Here's how the part is built. I have some questions about the finished solid (model axes, mm). Face numbers are marked on the shaded views. A direction names the side the tool comes from. Coordinates: 2 decimals unless noted, no trailing zeros. Order: outer loops, then holes, each group sorted by start corner. A loop starts at its lowest first (then second) coordinate and runs counter-clockwise, first axis right, second up. Notation, with made-up numbers: (60.25, 34.5) - (73.25, 34.5) arc R9 ccw to (73.25, 49.5) - close; hole circle Ø10 at (43, -8.5). An arc over 180 degrees is marked (long way). Answer as CSV lines item,"result". Start each with the question number.
Q1. For pin 1 Ø7.5 at (y, z) = (-3, 12) entering from +X; pin 2 Ø10 at (x, z) = (-19.5, 12.5) entering from +Y; pin 3 Ø2 at (x, y) = (26.5, -24) entering from +Z; pin 4 Ø2.5 at (x, z) = (4, 13) entering from -Y, each with a flat end and sliding along its axis, tell me the tip position at first contact or that it passes through.
Q2. Thinking about a two-plate mould opening in X: for the marked faces 6, 7, 8 and 9, which applies, released by +X, released by -X, zero draft, split by the parting line, or undercut?
Q3. Suppose I cut it at A-A (y = 0). Please give me the cut outline in (x, z) (3 decimals).
Q4. For the marked faces 1, 2, 3, 4 and 5, which set-ups out of +Z, -Z, +X, -X, +Y, -Y let a thin tool reach every point of the face, with its end or its side?
Q5. Suppose I cut it at B-B (z = 8.5). Please give me the cut outline in (x, y), then the cut area to 3 significant figures.
Q6. I need wall thicknesses on line 1 (X direction, y = 4, z = 5.5) (3 decimals); line 2 (X direction, y = -4, z = 12.5); line 3 (Z direction, x = -4, y = 0). Which ranges of each line are inside material? Lowest first, please.
Q7. Suppose I cut it at D-D (z = 20.5). Please give me the cut outline in (x, y).
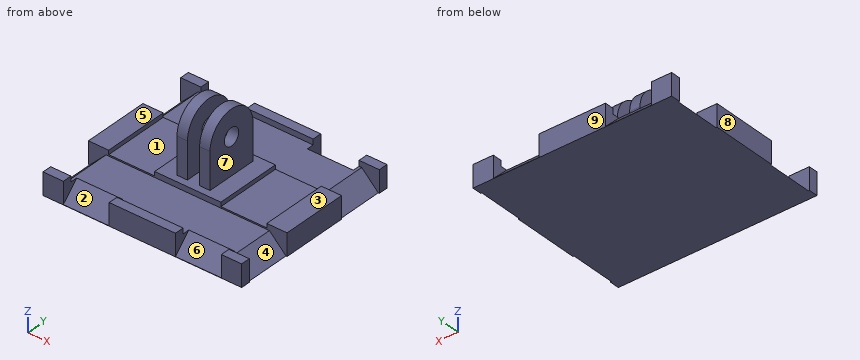
from build123d import *

# Parameters (mm, degrees)
F0_W         = 57.15
F0_H         = 50.8
F1_DEPTH     = 6.35
F2_W         = 13.208
F2_H         = 1.190625
F3_DEPTH     = 50.801
F4_SIZE      = 5.08
F5_W         = 3
F5_H         = 15
F6_DEPTH     = 18
F8_D         = 5
F9_W         = 13.208
F9_H         = 1.5875
F10_DEPTH    = 57.151
F11_T1_DEPTH = 13.208
F11_T3_DEPTH = 13.208
F13_DEPTH    = 33.326


# Not quite as in the source:
# - a fillet or chamfer that OpenCascade refuses, or shapes differently, is made with other operations: its cross-section is extruded or revolved along the edge and cut away or added


with BuildPart() as f1:
    # F0 (on Top) → F1 (new body)
    with BuildSketch(Plane.XY):
        Rectangle(F0_W, F0_H)
    extrude(amount=F1_DEPTH)

    # F2 (on face) → F3 (cut, through all)
    with BuildSketch(Plane.XZ.offset(25.4)):
        with Locations((-16.129, 5.7546875)):
            Rectangle(F2_W, F2_H)
        with Locations((16.129, 5.7546875)):
            Rectangle(F2_W, F2_H)
    extrude(amount=-F3_DEPTH, mode=Mode.SUBTRACT)

    # F4
    f4_edges = [f1.edges().sort_by_distance(p)[0] for p in [
        (-16.129, -25.4, 5.159375),
        (16.129, -25.4, 5.159375),
        (-16.129, 25.4, 5.159375),
        (16.129, 25.4, 5.159375),
    ]]
    chamfer(f4_edges, length=F4_SIZE)

    # F5 (on face) → F6 (join)
    with BuildSketch(Plane.XY.offset(6.35)):
        with Locations((-3.25, 0)):
            Rectangle(F5_W, F5_H)
        with Locations((3.25, 0)):
            Rectangle(F5_W, F5_H)
    extrude(amount=F6_DEPTH)

    # F8 (through all)
    with Locations(Plane.YZ.offset(4.75)):
        with Locations((0, 16.85)):
            Hole(F8_D / 2)

    # F9 (on face) → F10 (cut, through all)
    with BuildSketch(Plane.YZ.offset(28.575)):
        with Locations((-16.129, 5.55625)):
            Rectangle(F9_W, F9_H)
        with Locations((16.129, 5.55625)):
            Rectangle(F9_W, F9_H)
    extrude(amount=-F10_DEPTH, mode=Mode.SUBTRACT)

    # F11: chamfer of 5.08 on 4 edges, made by hand

    # F11_s2 → F11_t1 (cut)
    with BuildSketch(Plane.XZ.offset(-22.733)):
        Polygon((28.575, -0.3175), (23.495, 4.7625), (28.575, 4.7625), align=None)
        Polygon((-28.575, -0.3175), (-23.495, 4.7625), (-28.575, 4.7625), align=None)
    extrude(amount=F11_T1_DEPTH, mode=Mode.SUBTRACT)

    # F11_s4 → F11_t3 (cut)
    with BuildSketch(Plane.XZ.offset(9.525)):
        Polygon((28.575, -0.3175), (23.495, 4.7625), (28.575, 4.7625), align=None)
        Polygon((-28.575, -0.3175), (-23.495, 4.7625), (-28.575, 4.7625), align=None)
    extrude(amount=F11_T3_DEPTH, mode=Mode.SUBTRACT)

    # F12 (on face) → F13 (cut, through all)
    with BuildSketch(Plane(origin=(-4.75, 0, 0), x_dir=(0, -1, 0), z_dir=(-1, 0, 0))):
        with BuildLine():
            Line((-7.5, 24.35), (-7.5, 16.85))
            ThreePointArc((-7.5, 16.85), (-5.3033008589, 22.1533008589), (0, 24.35))
            Line((0, 24.35), (-7.5, 24.35))
        make_face()
        with BuildLine():
            Line((7.5, 24.35), (0, 24.35))
            ThreePointArc((0, 24.35), (5.3033008589, 22.1533008589), (7.5, 16.85))
            Line((7.5, 16.85), (7.5, 24.35))
        make_face()
    extrude(amount=-F13_DEPTH, mode=Mode.SUBTRACT)


solid = f1.part
Here are the results:
1,pin 1,"stops at x = 4.75"
1,pin 2,"passes through"
1,pin 3,"stops at z = 6.35"
1,pin 4,"stops at y = -7.5"
2,face 6,"undercut"
2,face 7,"released by +X"
2,face 8,"released by -X"
2,face 9,"zero draft"
3,outline,"(-28.575, 0) - (28.575, 0) - (28.575, 6.35) - (22.733, 6.35) - (22.733, 5.159) - (9.525, 5.159) - (9.525, 6.35) - (4.75, 6.35) - (4.75, 14.35) - (1.75, 14.35) - (1.75, 6.35) - (-1.75, 6.35) - (-1.75, 14.35) - (-4.75, 14.35) - (-4.75, 6.35) - (-9.525, 6.35) - (-9.525, 5.159) - (-22.733, 5.159) - (-22.733, 6.35) - (-28.575, 6.35) - close; (-4.75, 19.35) - (-1.75, 19.35) - (-1.75, 24.35) - (-4.75, 24.35) - close; (1.75, 19.35) - (4.75, 19.35) - (4.75, 24.35) - (1.75, 24.35) - close"
4,face 1,"+Z, +Y, -Y"
4,face 2,"+Z, -Y"
4,face 3,"+Z, +X, +Y, -Y"
4,face 4,"+Z, +X"
4,face 5,"+Z, -X, +Y, -Y"
5,outline,"(-4.75, -7.5) - (-1.75, -7.5) - (-1.75, 7.5) - (-4.75, 7.5) - close; (1.75, -7.5) - (4.75, -7.5) - (4.75, 7.5) - (1.75, 7.5) - close"
5,area,"90.0 mm²"
6,line 1,"x = -28.575 to -22.733, -9.525 to 9.525, 22.733 to 28.575"
6,line 2,"x = -4.75 to -1.75, 1.75 to 4.75"
6,line 3,"z = 0 to 14.35, 19.35 to 24.35"
7,outline,"(-4.75, -6.55) - (-1.75, -6.55) - (-1.75, 6.55) - (-4.75, 6.55) - close; (1.75, -6.55) - (4.75, -6.55) - (4.75, 6.55) - (1.75, 6.55) - close"
